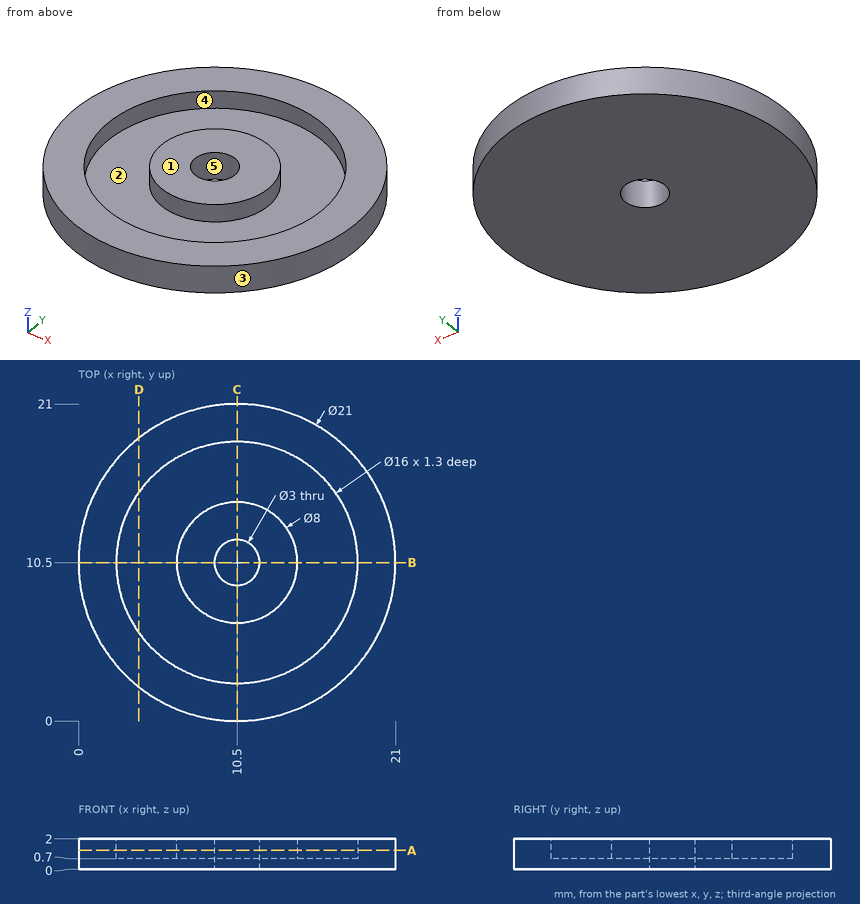
Geometry: see drawing. Coordinates: mm, zero at the bounding-box minimum. A direction names the side the tool comes from. Round coordinates to 2 decimals unless told otherwise and drop trailing zeros. Loops run counter-clockwise (first coordinate to the right, second up) from the corner with the lowest first, then second, coordinate; pieces in that order, holes last. Notation, with made-up numbers: M -30.75,6 L -14.75,6 A22 cw -14.75,23 Z; hole C 83,49 d5. An arc over 180 degrees is marked long. Use a Markdown table: item, result. Add a question column.
1. Section query A-A on z = 1.25. Return the cut outline in (x, y), then the cut area to 3 significant figures.
2. Line query: line 1 (Y direction, x = 10.5, z = 1); line 2 (Y direction, x = 10.5, z = 0.6); line 3 (X direction, y = 7.75, z = 1.7). Output: solid intervals per line, ascending.
3. Section query B-B on y = 10.5. Return the cut outline in (x, z).
4. Contact query for a flat-ended pin moving along its axis: P1, Ø1, axis at y = 13, z = 1.5, coming from the +X side. Output: stop coordinate, or through.
5. Section query D-D on x = 4. Return the cut outline in (y, z).
6. Mould query, pull axis X, two halves, no side actions, for the marked faces 1, 2 and 3. Classes: pulls with the +X half, pulls with the -X half, needs draft (parallel to the pull), parting line crosses it, or undercut.
7. Reachability of the marked faces 4 and 5 from +Z, -Z, +X, -X, +Y, -Y: full face, straight path, thin tool, end or side. Return the list, or none.
Reported:
| question | item | result |
|---|---|---|
| 1 | outline | C 10.5,10.5 d21; C 10.5,10.5 d8; hole C 10.5,10.5 d16; hole C 10.5,10.5 d3 |
| 1 | area | 188 mm² |
| 2 | line 1 | y = 0 to 2.5, 6.5 to 9, 12 to 14.5, 18.5 to 21 |
| 2 | line 2 | y = 0 to 9, 12 to 21 |
| 2 | line 3 | x = 0.37 to 2.99, 7.6 to 13.4, 18.01 to 20.63 |
| 3 | outline | M 0,0 L 9,0 L 9,2 L 6.5,2 L 6.5,0.7 L 2.5,0.7 L 2.5,2 L 0,2 Z; M 12,0 L 21,0 L 21,2 L 18.5,2 L 18.5,0.7 L 14.5,0.7 L 14.5,2 L 12,2 Z |
| 4 | P1 | stops at x = 20.81 |
| 5 | outline | M 2.25,0 L 18.75,0 L 18.75,2 L 15.16,2 L 15.16,0.7 L 5.84,0.7 L 5.84,2 L 2.25,2 Z |
| 6 | face 1 | needs draft |
| 6 | face 2 | undercut |
| 6 | face 3 | parting line crosses it |
| 7 | face 4 | +Z |
| 7 | face 5 | +Z, -Z |
